Check sheet for the modelled part. Datum: model origin and axes. Units: mm. A direction names the side the tool comes from. Coordinates: 2 decimals unless noted, no trailing zeros. Loops run counter-clockwise (first coordinate to the right, second up) from the corner with the lowest first, then second, coordinate; pieces in that order, holes last. Notation, with made-up numbers: M 10,74.25 L 57,74.25 A29 ccw 57,105.25 Z; hole C 7.5,83.5 d4. An arc over 180 degrees is marked long. Return JSON: item names as keys, results as strings.
from build123d import *

# Parameters (mm, degrees)
F0_W      = 125.1319237053
F0_H      = 67.682877183
F1_DEPTH  = 12.7
F2_W      = 125.1319237053
F2_H      = 67.682877183
F3_DEPTH  = 60.96
F4_W      = 65.4733031988
F4_H      = 14.4204068929
F5_DEPTH  = 60.96
F6_W      = 59.6586205065
F6_H      = 55.4480541825
F7_DEPTH  = 10.16
F8_DEPTH  = 5.08
F9_DEPTH  = 5.08
F10_W     = 125.1319237053
F10_H     = 50.2397883683
F11_DEPTH = 35.56
F12_W     = 125.1319237053
F12_H     = 20.1084222645
F13_DEPTH = 25.4
F14_W     = 125.1319237053
F14_H     = 8.8336318731
F15_DEPTH = 25.4
F16_W     = 125.1319237053
F16_H     = 6.1016352847
F17_DEPTH = 25.4
F19_D     = 21.59
F21_D     = 21.59


with BuildPart() as f1:
    # F0 (on Top) → F1 (new body)
    with BuildSketch(Plane.XY):
        with Locations((2.9073413461, -5.6983865798)):
            Rectangle(F0_W, F0_H)
    extrude(amount=F1_DEPTH)

    # F2 (on face) → F3 (join)
    with BuildSketch(Plane.XY.offset(12.7)):
        with Locations((2.9073413461, -5.6983865798)):
            Rectangle(F2_W, F2_H)
    extrude(amount=F3_DEPTH)

    # F4 (on face) → F5 (cut)
    with BuildSketch(Plane.XY.offset(73.66)):
        with Locations((32.7366515994, -32.3296217248)):
            Rectangle(F4_W, F4_H)
    extrude(amount=-F5_DEPTH, mode=Mode.SUBTRACT)

    # F6 (on face) → F7 (cut)
    with BuildSketch(Plane.XZ.offset(39.5398251712)):
        with Locations((-29.8293102533, 40.4240270913)):
            Rectangle(F6_W, F6_H)
    extrude(amount=-F7_DEPTH, mode=Mode.SUBTRACT)

    # F8 (add): a face of the model
    f8_faces = [f1.faces().sort_by_distance(p)[0] for p in [
        (32.7366515994, -25.1194182783, 43.18),
    ]]
    extrude(f8_faces, amount=F8_DEPTH)

    # F9 (cut): faces of the model
    f9_faces = [f1.faces().sort_by_distance(p)[0] for p in [
        (32.7366515994, -30.1994182783, 43.18),
        (-29.8293102533, -29.3798251712, 40.4240270913),
    ]]
    extrude(f9_faces, amount=-F9_DEPTH, mode=Mode.SUBTRACT)

    # F10 (on face) → F11 (cut)
    with BuildSketch(Plane(origin=(0, 28.1430520117, 0), x_dir=(-1, 0, 0), z_dir=(0, 1, 0))):
        with Locations((-2.9073413461, 37.1288014576)):
            Rectangle(F10_W, F10_H)
    extrude(amount=-F11_DEPTH, mode=Mode.SUBTRACT)

    # F12 (on face) → F13 (cut)
    with BuildSketch(Plane.XY.offset(12.0089072734)):
        with Locations((2.9073413461, 18.0888408795)):
            Rectangle(F12_W, F12_H)
    extrude(amount=-F13_DEPTH, mode=Mode.SUBTRACT)

    # F14 (on face) → F15 (cut)
    with BuildSketch(Plane.XY.offset(73.66)):
        with Locations((2.9073413461, 23.7262360752)):
            Rectangle(F14_W, F14_H)
    extrude(amount=-F15_DEPTH, mode=Mode.SUBTRACT)

    # F16 (on face) → F17 (cut)
    with BuildSketch(Plane.XY.offset(73.66)):
        with Locations((2.9073413461, 16.2586024962)):
            Rectangle(F16_W, F16_H)
    extrude(amount=-F17_DEPTH, mode=Mode.SUBTRACT)

    # F19 (through all)
    with Locations(Plane.XZ.offset(24.2998251712)):
        with Locations((-34.0740270913, 41.1679372191)):
            Hole(F19_D / 2)

    # F21 (through all)
    with Locations(Plane.XZ.offset(25.1194182783)):
        with Locations((33.1436805427, 40.4701754451)):
            Hole(F21_D / 2)


solid = f1.part
1) Section check A-A on y = 2. Record the cut outline in (x, z), then the cut area to 3 significant figures.
Answers:
{"outline": "M -59.66,0 L 65.47,0 L 65.47,12.01 L -59.66,12.01 Z; M -59.66,62.25 L 65.47,62.25 L 65.47,73.66 L -59.66,73.66 Z", "area": "2,930 mm²"}
2) Scan lines: line 1 along Z through (x, y) = (-10.5, -29); line 2 along X through (y, z) = (-9, 49); line 3 along Z through (x, y) = (-38, -5.5). Record each from-to range of solid material in increasing order. Write a range as [from, to].
Answers:
{"line 1": "[0, 12.7], [68.15, 73.66]", "line 2": "[-59.66, -41.5], [-26.64, 26.53], [39.76, 65.47]", "line 3": "[0, 12.01], [62.25, 73.66]"}
3) Set-up check for faces 5 (the face through (4, 3, 62.249)), 6 (the face through (-24, -24.3, 35)), 7 (the face through (0, -32, 71)): record each of +Z, -Z, +X, -X, +Y, -Y from which the full face is reachable in a straight line by a thin tool's end or side.
Answers:
{"face 5": "+X, -X, +Y", "face 6": "-X, -Y", "face 7": "+Z, +X, -Y"}
4) Section check D-D on y = -29.5. Record the cut outline in (x, z).
Answers:
{"outline": "M -59.66,0 L 65.47,0 L 65.47,12.7 L -59.66,12.7 Z; M -59.66,68.15 L 0,68.15 L 0,73.66 L -59.66,73.66 Z"}
5) Section check B-B on x = -25.5. Record the cut outline in (y, z).
Answers:
{"outline": "M -39.54,0 L 8.03,0 L 8.03,12.01 L -7.42,12.01 L -7.42,34.61 L -24.3,34.61 L -24.3,12.7 L -39.54,12.7 Z; M -39.54,68.15 L -24.3,68.15 L -24.3,47.73 L -7.42,47.73 L -7.42,62.25 L 13.21,62.25 L 13.21,73.66 L -39.54,73.66 Z"}
6) Go/stop test with flat-tipped pins: pin 1 Ø2 at (x, z) = (-33.5, 24) entering from -Y; pin 2 Ø1.7 at (y, z) = (-34.5, 71) entering from +X; pin 3 Ø4.5 at (x, y) = (13.5, -33.5) entering from +Z. Record where each tip stops, or that it passes through.
Answers:
{"pin 1": "y = -24.3", "pin 2": "x = 0", "pin 3": "z = 12.7"}
7) Draft check along Z on faces 1 (the face through (2, -13, 73.66)), 2 (the face through (-31.73, -15.74, 30.63)), 3 (the face through (2, -39.54, 6)), 4 (the face through (4, 0, 12.009)). Enter one of: +Z half, -Z half, draft (parallel to the pull), parting line (faces both ways), or undercut.
Answers:
{"face 1": "+Z half", "face 2": "undercut", "face 3": "draft", "face 4": "undercut"}
8) Section check C-C on z = 46.5. Record the cut outline in (x, y), then the cut area to 3 significant figures.
Answers:
{"outline": "M -59.66,-24.3 L -43.46,-24.3 L -43.46,-7.42 L -59.66,-7.42 Z; M -24.69,-24.3 L 0,-24.3 L 0,-25.12 L 24.19,-25.12 L 24.19,-7.42 L -24.69,-7.42 Z; M 42.1,-25.12 L 65.47,-25.12 L 65.47,-7.42 L 42.1,-7.42 Z", "area": "1,530 mm²"}
